```python
from build123d import *

# Parameters (mm, degrees)
SKETCH_1_W                         = 114
SKETCH_1_H                         = 15
EXTRUDE_1_DEPTH                    = 1
SM_EDGE_FLANGE_1_STRIP_W           = 5
SM_EDGE_FLANGE_1_STRIP_H           = 1
SM_EDGE_FLANGE_1_STRIP_CUT_DEPTH   = 15
SM_EDGE_FLANGE_1_STRIP_2_W         = 5
SM_EDGE_FLANGE_1_STRIP_2_H         = 1
SM_EDGE_FLANGE_1_STRIP_CUT_2_DEPTH = 15
SM_EDGE_FLANGE_1_DEPTH             = 15
SM_EDGE_FLANGE_1_BEND_DEPTH        = 15
CUT_EXTRUDE_1_DEPTH                = 58.630287176
SKETCH_13_R                        = 1.5
CUT_EXTRUDE_2_DEPTH                = 5
FILLET_1_R                         = 2


# Sheet-metal steps are written as plain solids
with BuildPart() as part:
    # Sketch 1 → Бобышка-Вытянуть1 (new body)
    with BuildSketch(Plane(origin=(0, 0, 0), x_dir=(1, 0, 0), z_dir=(0, 1, 0))):
        Rectangle(SKETCH_1_W, SKETCH_1_H)
    extrude(amount=EXTRUDE_1_DEPTH)

    # Ребро-кромка1 strip (across the edge) → Ребро-кромка1 strip cut (cut)
    with BuildSketch(Plane(origin=(57, 1, 7.5), x_dir=(-1, 0, 0), z_dir=(0, 0, -1))):
        with Locations((-1, -0.5)):
            Rectangle(SM_EDGE_FLANGE_1_STRIP_W, SM_EDGE_FLANGE_1_STRIP_H)
    extrude(amount=SM_EDGE_FLANGE_1_STRIP_CUT_DEPTH, mode=Mode.SUBTRACT)

    # Ребро-кромка1 strip 2 (across the edge) → Ребро-кромка1 strip cut 2 (cut)
    with BuildSketch(Plane(origin=(-57, 1, -7.5), x_dir=(1, 0, 0), z_dir=(0, 0, 1))):
        with Locations((-1, -0.5)):
            Rectangle(SM_EDGE_FLANGE_1_STRIP_2_W, SM_EDGE_FLANGE_1_STRIP_2_H)
    extrude(amount=SM_EDGE_FLANGE_1_STRIP_CUT_2_DEPTH, mode=Mode.SUBTRACT)

    # Ребро-кромка1 section (across the edge) → Ребро-кромка1 (add)
    with BuildSketch(Plane(origin=(57, 1, 7.5), x_dir=(-1, 0, 0), z_dir=(0, 0, -1))):
        with BuildLine():
            Line((0, 0.5), (0, 4))
            Line((0, 4), (1, 4))
            Line((1, 4), (1, 0.5))
            ThreePointArc((1, 0.5), (1.146446609, 0.146446609), (1.5, 0))
            Line((1.5, 0), (1.5, -1))
            ThreePointArc((1.5, -1), (0.439339828, -0.560660172), (0, 0.5))
        make_face()
    extrude(amount=SM_EDGE_FLANGE_1_DEPTH)

    # Ребро-кромка1 section 2 (across the edge) → Ребро-кромка1 bend (add)
    with BuildSketch(Plane(origin=(-57, 1, -7.5), x_dir=(1, 0, 0), z_dir=(0, 0, 1))):
        with BuildLine():
            Line((0, 0.5), (0, 4))
            Line((0, 4), (1, 4))
            Line((1, 4), (1, 0.5))
            ThreePointArc((1, 0.5), (1.146446609, 0.146446609), (1.5, 0))
            Line((1.5, 0), (1.5, -1))
            ThreePointArc((1.5, -1), (0.439339828, -0.560660172), (0, 0.5))
        make_face()
    extrude(amount=SM_EDGE_FLANGE_1_BEND_DEPTH)

    # Эскиз12 → Вырез-Вытянуть1 (cut, through all)
    with BuildSketch(Plane(origin=(0, 1, 0), x_dir=(1, 0, 0), z_dir=(0, 1, 0))):
        with BuildLine():
            Line((-20, 1.5), (-13, 1.5))
            ThreePointArc((-13, 1.5), (-11.5, 0), (-13, -1.5))
            Line((-13, -1.5), (-20, -1.5))
            ThreePointArc((-20, -1.5), (-21.5, 0), (-20, 1.5))
        make_face()
        with BuildLine():
            Line((20, 1.5), (13, 1.5))
            ThreePointArc((13, 1.5), (11.5, 0), (13, -1.5))
            Line((13, -1.5), (20, -1.5))
            ThreePointArc((20, -1.5), (21.5, 0), (20, 1.5))
        make_face()
    extrude(amount=-CUT_EXTRUDE_1_DEPTH, mode=Mode.SUBTRACT)

    # Эскиз13 → Вырез-Вытянуть2 (cut)
    with BuildSketch(Plane(origin=(0, 1, 0), x_dir=(1, 0, 0), z_dir=(0, 1, 0))):
        with Locations(Location((-49, 0, 0), (0, 0, 270))):
            Circle(SKETCH_13_R)
        with Locations(Location((49, 0, 0), (0, 0, 270))):
            Circle(SKETCH_13_R)
    extrude(amount=-CUT_EXTRUDE_2_DEPTH, mode=Mode.SUBTRACT)

    # Скругление1
    fillet_1_edges = [part.edges().sort_by_distance(p)[0] for p in [
        (56.5, 5, 7.5),
        (56.5, 5, -7.5),
        (-56.5, 5, -7.5),
        (-56.5, 5, 7.5),
    ]]
    fillet(fillet_1_edges, radius=FILLET_1_R)


solid = part.part
```
Geometry check sheet. Reference: the model listing, model coordinates, mm. A direction names the side the tool comes from. Give positions to 0.01 mm unless a question says otherwise; leave off trailing zeros. Order: outer loops, then holes, each group sorted by start corner. A loop starts at its lowest first (then second) coordinate and runs counter-clockwise, first axis right, second up. Notation, with made-up numbers: (18, 51) - (31, 51) arc R18 ccw to (31, 62) - close; hole circle Ø7 at (-29.5, 66.5). An arc over 180 degrees is marked (long way). Write item = value, one per line. Start each with the question number.
1) Gauge pin test, flat ends, axial feed: pin 1 Ø4 at (x, z) = (-41, -2.5) entering from +Y; pin 2 Ø1.8 at (x, z) = (-49, 0) entering from +Y. Record the tip position at first contact, or that the pin passes through.
2) Section check B-B (x = 49). Enter the section's corners in (y, z), then the cut area to 3 significant figures.
3) Section check A-A (z = 0). Enter the section's corners in (x, y).
4) Section check C-C (x = 24). Enter the section's corners in (y, z).
5) Access from +Z, -Z, +X, -X, +Y, -Y to the whole of each face (thin tool, end or side, straight path). Record for faces 4 (the flat face through (-1, 1, 0)), 5 (the cylindrical face through (-56.49, 4.43, -6.9)).
6) Scan lines: L1, parallel to X at y = 1.4, z = 0.5; L2, parallel to X at y = 0.3, z = 0; L3, parallel to Y at x = 17.5, z = -1.75. Record each from-to range of solid material in increasing order.
7) Draft check along X on faces 1 (the cylindrical face through (56.49, 4.4, 6.93)), 2 (the flat face through (-56, 3, 0)), 3 (the flat face through (-57, 3, 0)). Enter one of: released by +X, released by -X, zero draft, split by the parting line, or undercut.
Geometry check:
q1.pin_1 = 1
q1.pin_2 = through
q2.outline = (0, -7.5) - (1, -7.5) - (1, -1.5) - (0, -1.5) - close; (0, 1.5) - (1, 1.5) - (1, 7.5) - (0, 7.5) - close
q2.area = 12.0 mm2
q3.outline = (-57, 1.5) arc R1.5 ccw to (-55.5, 0) - (-50.5, 0) - (-50.5, 1) - (-55.5, 1) arc R0.5 cw to (-56, 1.5) - (-56, 5) - (-57, 5) - close; (-47.5, 0) - (-21.5, 0) - (-21.5, 1) - (-47.5, 1) - close; (-11.5, 0) - (11.5, 0) - (11.5, 1) - (-11.5, 1) - close; (21.5, 0) - (47.5, 0) - (47.5, 1) - (21.5, 1) - close; (50.5, 0) - (55.5, 0) arc R1.5 ccw to (57, 1.5) - (57, 5) - (56, 5) - (56, 1.5) arc R0.5 cw to (55.5, 1) - (50.5, 1) - close
q4.outline = (0, -7.5) - (1, -7.5) - (1, 7.5) - (0, 7.5) - close
q5.face_4 = +Z, -Z, +Y
q5.face_5 = -Z, +X, -X, +Y
q6.L1 = -57 to -55.99, 55.99 to 57
q6.L2 = -56.4 to -50.5, -47.5 to -21.5, -11.5 to 11.5, 21.5 to 47.5, 50.5 to 56.4
q6.L3 = 0 to 1
q7.face_1 = zero draft
q7.face_2 = undercut
q7.face_3 = released by -X
